Can you work these out from the model? Positions are in its coordinate system, mm. Face numbers are marked on the shaded views. A direction names the side the tool comes from. Give positions to 0.01 mm unless a question says otherwise; leave off trailing zeros. Loops run counter-clockwise (first coordinate to the right, second up) from the corner with the lowest first, then second, coordinate; pieces in that order, holes last.
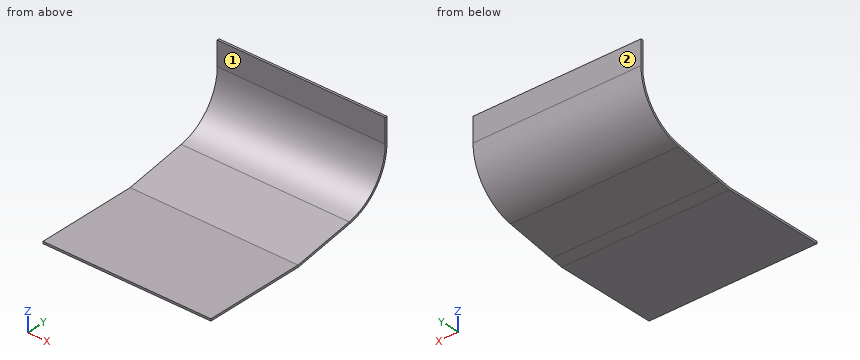
from build123d import *

# Parameters (mm, degrees)
F1_DEPTH = 127


with BuildPart() as f1:
    # F0 (on Right) → F1 (new body)
    with BuildSketch(Plane.YZ):
        with BuildLine():
            Line((120.915996, 7.884636), (76.2, 0))
            Line((76.2, 0), (85.342048, 0))
            Line((85.342048, 0), (121.191662, 6.321254))
            ThreePointArc((121.191662, 6.321254), (144.702389, 19.895179), (153.9875, 45.405812))
            Line((153.9875, 45.405812), (153.9875, 63.5))
            Line((153.9875, 63.5), (152.4, 63.5))
            Line((152.4, 63.5), (152.4, 45.405812))
            ThreePointArc((152.4, 45.405812), (143.486293, 20.915604), (120.915996, 7.884636))
        make_face()
        Polygon((76.2, 0), (0, 0), (0, -1.5875), (76.338888, -1.5875), (85.342048, 0), align=None)
    extrude(amount=F1_DEPTH)


solid = f1.part
(1) Suppose I cut it at C-C on y = 38. List the corners of the cut face in (x, z) for me, plus the area to 3 significant figures.
Returned:
outline: (0, -1.59) - (127, -1.59) - (127, 0) - (0, 0) - close
area: 202 mm2
(2) Which directions (+Z, -Z, +X, -X, +Y, -Y) give clear straight access to the entire face, cutting with the end or side of a thin tool? Please do the marked faces 1 and 2.
Returned:
face 1: +Z, +X, -X, -Y
face 2: +Z, -Z, +X, -X, +Y
(3) Suppose I cut it at A-A on x = 110. List the corners of the cut face in (y, z) for me (1 decimal), plus the area to 3 significant figures.
Returned:
outline: (0, -1.6) - (76.3, -1.6) - (121.2, 6.3) arc R39.7 ccw to (154, 45.4) - (154, 63.5) - (152.4, 63.5) - (152.4, 45.4) arc R38.1 cw to (120.9, 7.9) - (76.2, 0) - (0, 0) - close
area: 308 mm2
(4) Will these pins go through, and if not, where does the flat tip stop? P1, Ø23, axis at x = 74.5, y = 38, coming from the +Z side; P2, Ø4, axis at x = 105, z = 37.5, coming from the +Y side; P3, Ø9, axis at x = 58, z = 57, coming from the -Y side.
Returned:
P1: stops at z = 0
P2: stops at y = 153.55
P3: stops at y = 152.4
(5) Please list where these lines run through material, in increasing order: probe 1 along Y at (x, z) = (68, 46); probe 2 along Z at (x, y) = (48.5, 16.5); probe 3 along Y at (x, z) = (105.5, 33.5).
Returned:
probe 1: y = 152.4 to 153.99
probe 2: z = -1.59 to 0
probe 3: y = 150.49 to 152.16
(6) Suppose I cut it at B-B on z = 52.5. List the corners of the cut face in (x, y) for me.
Returned:
outline: (0, 152.4) - (127, 152.4) - (127, 153.99) - (0, 153.99) - close
